Check sheet for the modelled part. Datum: model origin and axes. Units: mm. Face numbers are marked on the shaded views. A direction names the side the tool comes from. Give positions to 0.01 mm unless a question says otherwise; leave off trailing zeros. Order: outer loops, then holes, each group sorted by start corner. A loop starts at its lowest first (then second) coordinate and runs counter-clockwise, first axis right, second up.
```python
from build123d import *

# Parameters (mm, degrees)
BOSS_EXTRUDE1_DEPTH                         = 8
FILLET1_R                                   = 12
FILLET2_R                                   = 5
FILLET3_R                                   = 5
CHAMFER2_SIZE                               = 1
F_5_0MM_DOWEL_HOLE3_D                       = 5
F_3_0MM_DOWEL_HOLE1_D                       = 3
CBORE_FOR_M5_CHEESE_HEAD_SCREW5_D           = 5.5
CBORE_FOR_M5_CHEESE_HEAD_SCREW5_CBORE_D     = 10
CBORE_FOR_M5_CHEESE_HEAD_SCREW5_CBORE_DEPTH = 3.3
CBORE_FOR_M5_CHEESE_HEAD_SCREW6_D           = 5.5
CBORE_FOR_M5_CHEESE_HEAD_SCREW6_CBORE_D     = 10
CBORE_FOR_M5_CHEESE_HEAD_SCREW6_CBORE_DEPTH = 3.3
F_8_0MM_DOWEL_HOLE3_D                       = 8


with BuildPart() as part:
    # Sketch1 → Boss-Extrude1 (new body)
    with BuildSketch(Plane(origin=(0, 0, 0), x_dir=(0, 0, -1), z_dir=(1, 0, 0))):
        Polygon((65, 0), (65, 45), (46.983473404, 94.5), (0, 94.5), (0, 71.5), (20, 71.5), (20, 48.5), (10, 48.5), (10, 0), align=None)
    extrude(amount=BOSS_EXTRUDE1_DEPTH)

    # Fillet1
    fillet1_edges = [part.edges().sort_by_distance(p)[0] for p in [
        (4, 94.5, -46.983473404),
    ]]
    fillet(fillet1_edges, radius=FILLET1_R)

    # Fillet2
    fillet2_edges = [part.edges().sort_by_distance(p)[0] for p in [
        (4, 94.5, 0),
    ]]
    fillet(fillet2_edges, radius=FILLET2_R)

    # Fillet3
    fillet3_edges = [part.edges().sort_by_distance(p)[0] for p in [
        (4, 48.5, -20),
        (4, 71.5, -20),
    ]]
    fillet(fillet3_edges, radius=FILLET3_R)
    fillet3_2_edges = [part.edges().sort_by_distance(p)[0] for p in [
        (4, 48.5, -10),
        (4, 71.5, 0),
    ]]
    fillet(fillet3_2_edges, radius=FILLET3_R - 0.0001)  # a hair under: the kernel refuses the full size

    # Chamfer2
    chamfer2_edges = [part.edges().sort_by_distance(p)[0] for p in [
        (4, 0, -65),
        (4, 0, -10),
    ]]
    chamfer(chamfer2_edges, length=CHAMFER2_SIZE)

    # Ø5.0mm Dowel Hole3 (through all)
    with Locations(Plane(origin=(0, 0, 0), x_dir=(0, 0, -1), z_dir=(-1, 0, 0))):
        with Locations((40, -35), (40, -10.001113523)):
            Hole(F_5_0MM_DOWEL_HOLE3_D / 2)

    # Ø3.0mm Dowel Hole1 (through all)
    with Locations(Plane(origin=(0, 0, 0), x_dir=(0, 0, -1), z_dir=(-1, 0, 0))):
        with Locations((39.239701592, -22)):
            Hole(F_3_0MM_DOWEL_HOLE1_D / 2)

    # CBORE for M5 Cheese Head Screw5 (through all)
    with Locations(Plane(origin=(8, 0, 0), x_dir=(0, 0, -1), z_dir=(1, 0, 0))):
        with Locations((30, 10.001113523)):
            CounterBoreHole(CBORE_FOR_M5_CHEESE_HEAD_SCREW5_D / 2, CBORE_FOR_M5_CHEESE_HEAD_SCREW5_CBORE_D / 2, CBORE_FOR_M5_CHEESE_HEAD_SCREW5_CBORE_DEPTH)

    # CBORE for M5 Cheese Head Screw6 (through all)
    with Locations(Plane(origin=(8, 0, 0), x_dir=(0, 0, -1), z_dir=(1, 0, 0))):
        with Locations((50.552772121, 35)):
            CounterBoreHole(CBORE_FOR_M5_CHEESE_HEAD_SCREW6_D / 2, CBORE_FOR_M5_CHEESE_HEAD_SCREW6_CBORE_D / 2, CBORE_FOR_M5_CHEESE_HEAD_SCREW6_CBORE_DEPTH)

    # Ø8.0mm Dowel Hole3 (through all)
    with Locations(Plane(origin=(0, 0, 0), x_dir=(0, 0, -1), z_dir=(-1, 0, 0))):
        with Locations((24.5, -82)):
            Hole(F_8_0MM_DOWEL_HOLE3_D / 2)


solid = part.part
```
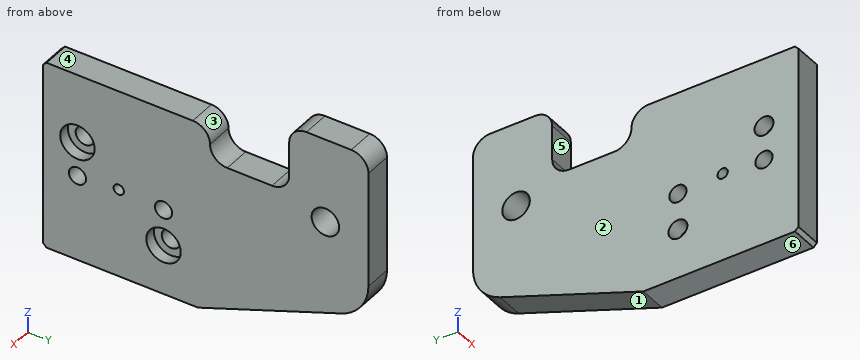
(1) Material ranges on L1, parallel to Y at x = 7.1, z = -30; L2, parallel to Y at x = 5.5, z = -40; L3, parallel to Y at x = 2.9, z = -30, recorded low to high.
Response values:
L1: y = 0 to 5, 15 to 94.5
L2: y = 0 to 7.5, 12.5 to 20.71, 23.29 to 32.5, 37.5 to 94.42
L3: y = 0 to 7.25, 12.75 to 94.5
(2) Cross-section at C-C on y = 22. Enter the section's corners in (x, z), then the cut area to 3 significant figures.
Response values:
outline: (0, -65) - (8, -65) - (8, -40.74) - (0, -40.74) - close; (0, -37.74) - (8, -37.74) - (8, -10) - (0, -10) - close
area: 416 mm2
(3) Gauge pin test, flat ends, axial feed: pin 1 Ø4 at (x, y) = (4.5, 58) entering from +Z; pin 2 Ø2.5 at (x, y) = (4, 26.5) entering from +Z; pin 3 Ø3 at (y, z) = (37.5, -51) entering from +X. Record the tip position at first contact, or that the pin passes through.
Response values:
pin 1: stops at z = -20
pin 2: stops at z = -10
pin 3: stops at x = 4.7
(4) Release check for a two-part mould opening along Y. For the marked faces 1, 2 and 3 record: released by +Y, released by -Y, zero draft, split by the parting line, or undercut.
Response values:
face 1: released by +Y
face 2: zero draft
face 3: undercut
(5) Set-up check for the marked faces 4, 5 and 6: record each of +Z, -Z, +X, -X, +Y, -Y from which the full face is reachable in a straight line by a thin tool's end or side.
Response values:
face 4: +Z, +X, -X, -Y
face 5: +Z, +X, -X
face 6: -Z, +X, -X, +Y, -Y
(6) Cross-section at D-D on x = 3.5. Count the separate pieces of the cut face and the enclosed holes in it, then the cut area to 3 significant figures.
Response values:
separate pieces: 1
enclosed holes: 6
area: 4,590 mm2
(7) Cross-section at A-A on y = 35. Enter the section's corners in (x, z), then the cut area to 3 significant figures.
Response values:
outline: (0, -65) - (8, -65) - (8, -55.55) - (4.7, -55.55) - (4.7, -53.3) - (0, -53.3) - close; (0, -47.8) - (4.7, -47.8) - (4.7, -45.55) - (8, -45.55) - (8, -42.5) - (0, -42.5) - close; (0, -37.5) - (8, -37.5) - (8, -10) - (0, -10) - close
area: 341 mm2
(8) Cross-section at B-B on z = -30. Enter the section's corners in (x, y).
Response values:
outline: (0, 0) - (8, 0) - (8, 5) - (4.7, 5) - (4.7, 7.25) - (0, 7.25) - close; (0, 12.75) - (4.7, 12.75) - (4.7, 15) - (8, 15) - (8, 94.5) - (0, 94.5) - close
